from build123d import *

# Parameters (mm, degrees)
SKETCH1_W               = 13
SKETCH1_H               = 8
BOSS_EXTRUDE1_DEPTH     = 3
CUT_EXTRUDE1_DEPTH      = 16.556349186
CUT_EXTRUDE1_DEPTH_BACK = 16.556349186
CUT_EXTRUDE2_DEPTH      = 16.556349186
CUT_EXTRUDE2_DEPTH_BACK = 16.556349186
SKETCH4_R               = 1.8
CUT_EXTRUDE3_DEPTH      = 0.8
SKETCH5_W               = 8
SKETCH5_H               = 1
BOSS_EXTRUDE2_DEPTH     = 2
FILLET1_R               = 4
CUT_EXTRUDE4_DEPTH      = 0.4


with BuildPart() as part:
    # Sketch1 → Boss-Extrude1 (new body)
    with BuildSketch(Plane(origin=(0, 0, 0), x_dir=(1, 0, 0), z_dir=(0, 1, 0))):
        with Locations((6.5, 4)):
            Rectangle(SKETCH1_W, SKETCH1_H)
    extrude(amount=BOSS_EXTRUDE1_DEPTH)

    # Sketch2 → Cut-Extrude1 (cut, two sides: drawn at the far end of the back side and taken through both)
    with BuildSketch(Plane.XY.offset(-CUT_EXTRUDE1_DEPTH_BACK)):
        Polygon((0, 0), (0.6, 3), (0, 3), align=None)
        Polygon((13, 0), (12.4, 3), (13, 3), align=None)
    extrude(amount=CUT_EXTRUDE1_DEPTH + CUT_EXTRUDE1_DEPTH_BACK, mode=Mode.SUBTRACT)

    # Sketch3 → Cut-Extrude2 (cut, two sides: drawn at the far end of the back side and taken through both)
    with BuildSketch(Plane(origin=(0, 0, 0), x_dir=(0, 0, -1), z_dir=(1, 0, 0)).offset(-CUT_EXTRUDE2_DEPTH_BACK)):
        Polygon((0, 0), (0.6, 3), (0, 3), align=None)
        Polygon((8, 3), (7.4, 3), (8, 0), align=None)
    extrude(amount=CUT_EXTRUDE2_DEPTH + CUT_EXTRUDE2_DEPTH_BACK, mode=Mode.SUBTRACT)

    # Sketch4 → Cut-Extrude3 (cut)
    with BuildSketch(Plane.XZ):
        with Locations(Location((6.50000125, -3.75, 0), (0, 0, 270))):
            Circle(SKETCH4_R)
    extrude(amount=-CUT_EXTRUDE3_DEPTH, mode=Mode.SUBTRACT)

    # Sketch5 → Boss-Extrude2 (add)
    with BuildSketch(Plane.XZ):
        with Locations((6.500011, -7.5)):
            Rectangle(SKETCH5_W, SKETCH5_H)
    extrude(amount=BOSS_EXTRUDE2_DEPTH)

    # Fillet1
    # the kernel refuses this fillet: 4 mm, written as the material it takes off along each edge
    with BuildSketch(Plane(origin=(10.500011, -2, -16.660254038), x_dir=(0, 1, 0), z_dir=(0, 0, 1)), Plane(origin=(2.500011, -2, 1.660254038), x_dir=(0, 1, 0), z_dir=(0, 0, -1))) as fillet1_piece_1:
        with BuildLine():
            CenterArc((4, 3.464101615), FILLET1_R, 180, 60)
            Line((0, 3.464101615), (-0.08, 3.464101615))
            Line((-0.08, 3.464101615), (-0.08, 0))
            Line((-0.08, 0), (0, -0.08))
            ThreePointArc((0, -0.08), (1, -0.08), (1.96, -0.069282032))
            Line((1.96, -0.069282032), (2, 0))
        make_face()
    extrude(amount=18.320508076, mode=Mode.SUBTRACT)

    # Sketch6 → Cut-Extrude4 (cut)
    with BuildSketch(Plane(origin=(0, 3, 0), x_dir=(1, 0, 0), z_dir=(0, 1, 0))):
        Polygon((4.028737707, 2.518536397), (4.028737707, 5.518536397), (6.067199245, 5.518536397), (6.067199245, 5.018536397), (4.605660784, 5.018536397), (4.605660784, 4.287767167), (5.874891553, 4.287767167), (5.874891553, 3.787767167), (4.605660784, 3.787767167), (4.605660784, 2.518536397), align=None)
        Polygon((6.567199245, 2.518536397), (6.567199245, 5.518536397), (7.169963668, 5.518536397), (8.374891553, 3.546180628), (8.374891553, 5.518536397), (8.95181463, 5.518536397), (8.95181463, 2.518536397), (8.330420399, 2.518536397), (7.144122322, 4.459642167), (7.144122322, 2.518536397), align=None)
    extrude(amount=-CUT_EXTRUDE4_DEPTH, mode=Mode.SUBTRACT)


solid = part.part
Geometry check sheet. Reference: the model listing, model coordinates, mm. A direction names the side the tool comes from. Give positions to 0.01 mm unless a question says otherwise; leave off trailing zeros. Order: outer loops, then holes, each group sorted by start corner. A loop starts at its lowest first (then second) coordinate and runs counter-clockwise, first axis right, second up.
1) Draft check along Z on faces 4 (the flat face through (7, 0.8, -4)), 5 (the flat face through (0.3, 1.5, -4.1)), 6 (the flat face through (6.4, 1.5, -0.3)). Enter one of: released by +Z, released by -Z, zero draft, split by the parting line, or undercut.
Results are:
face 4: undercut
face 5: zero draft
face 6: released by +Z
2) Cross-section at A-A (y = 0.2). Record the boundary of the cut face in (x, z).
Results are:
outline: (0.04, -7.96) - (12.96, -7.96) - (12.96, -0.04) - (0.04, -0.04) - close; hole circle Ø3.6 at (6.5, -3.75)
3) Cross-section at C-C (x = 2.75). Record the boundary of the cut face in (y, z).
Results are:
outline: (-0.38, -8) - (0, -8) - (3, -7.4) - (3, -0.6) - (0, 0) - (0, -7) - (-0.38, -7) - close
4) Gauge pin test, flat ends, axial feed: pin 1 (1.6 mm diameter, centred on x = 7.5, y = -0.5, fed in from +Z); pin 2 (3 mm diameter, centred on x = 6.5, z = -3.5, fed in from -Y); pin 3 (1.5 mm diameter, centred on x = 11, z = -5.5, fed in from -Y). Record the tip position at first contact, or that the pin passes through.
Results are:
pin 1: stops at z = 0
pin 2: stops at y = 0.8
pin 3: stops at y = 0
5) Cross-section at D-D (y = 1.9). Record the boundary of the cut face in (x, z), then the cut area to 3 significant figures.
Results are:
outline: (0.38, -7.62) - (12.62, -7.62) - (12.62, -0.38) - (0.38, -0.38) - close
area: 88.6 mm2
6) Cross-section at B-B (z = -7.25). Record the boundary of the cut face in (x, y).
Results are:
outline: (0, 0) - (2.5, 0) arc R4 ccw to (5.96, -2) - (7.04, -2) arc R4 ccw to (10.5, 0) - (13, 0) - (12.4, 3) - (0.6, 3) - close
7) Material ranges on probe 1 along Z at (x, y) = (7.25, -0.15); probe 2 along X at (y, z) = (0.65, -3.75); probe 3 along X at (y, z) = (0.2, -3.75), recorded low to high.
Results are:
probe 1: z = -8 to -7
probe 2: x = 0.13 to 4.7, 8.3 to 12.87
probe 3: x = 0.04 to 4.7, 8.3 to 12.96
8) Tool access check on faces 1 (the flat face through (6, -1, -7)), 2 (the cylindrical face through (5.811, 0.394, -5.413)), 3 (the flat face through (7.76, 2.8, -4.55)). Record the directions out of +Z, -Z, +X, -X, +Y, -Y that give a thin tool (end or side, any length) a straight path to the whole face; none if there is none.
Results are:
face 1: +Z, +X, -X, -Y
face 2: -Y
face 3: +Y
